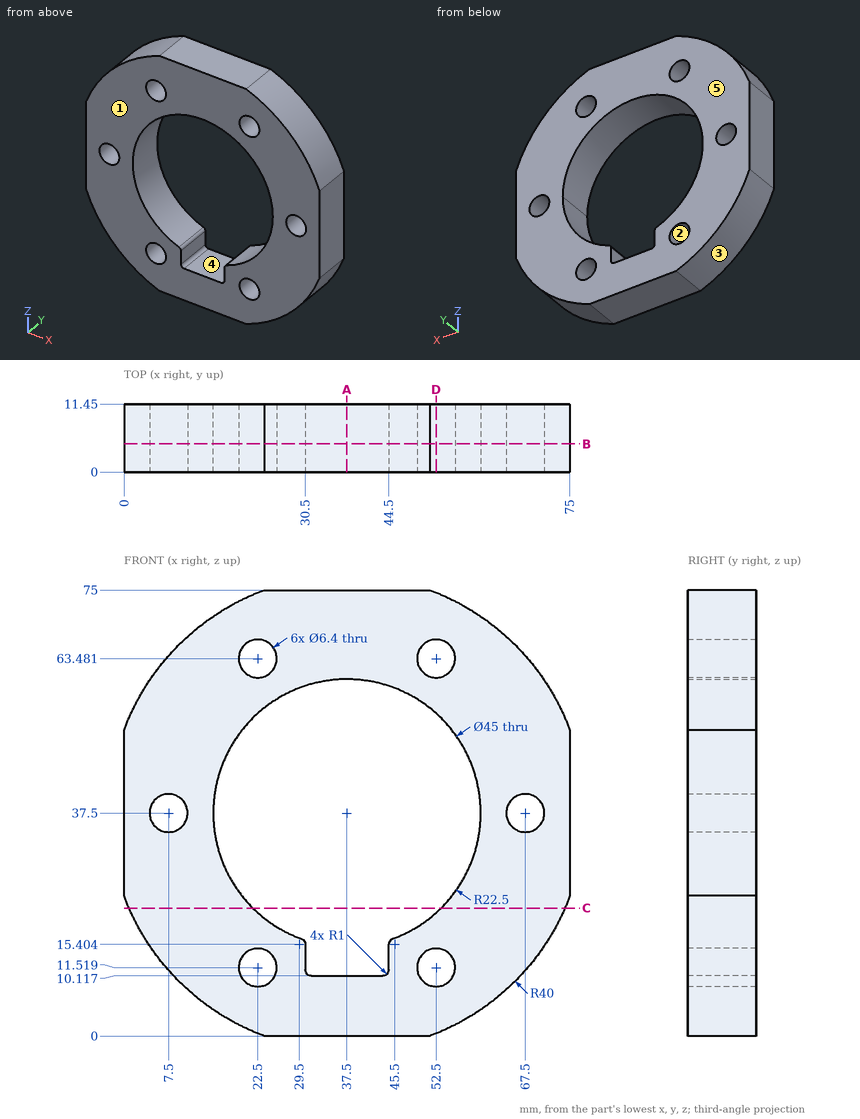
Source: three-view drawing plus pictorial views. Frame: mm from the lowest corner of the part. A direction names the side the tool comes from. Coordinates: 2 decimals unless noted, no trailing zeros. Loops run counter-clockwise (first coordinate to the right, second up) from the corner with the lowest first, then second, coordinate; pieces in that order, holes last. Notation, with made-up numbers: (42, -16) -> (68, -16) arc R13 cw to (68, 4) -> close; hole circle Ø10 at (64.25, 70). An arc over 180 degrees is marked (long way). Answer in a Markdown table with one row per item. Add a question column.
Q1. Ray query, line 1 along X through (y, z) = (2.5, 37.5); line 2 along X through (y, z) = (7.5, 61); line 3 along X through (y, z) = (1, 62) (1 decimal). Return the intervals inside material, ascending.
Q2. Section B-B on y = 4.75. Return the cut outline in (x, z), and give its area (3 significant figures).
Q3. Section C-C on z = 21.5. Return the cut outline in (x, y).
Q4. Section D-D on x = 52.5. Return the cut outline in (y, z).
Q5. Pull-direction query (Z, two-part tool) for the marked faces 1, 2 and 3; classes: pulls with the +Z half, pulls with the -Z half, needs draft (parallel to the pull), parting line crosses it, or undercut.
Q6. Reachability of the marked faces 4 and 5 from +Z, -Z, +X, -X, +Y, -Y: full face, straight path, thin tool, end or side. Return the list, or none.
Q7. Section A-A on x = 37.5. Return the cut outline in (y, z).
Q8. Contact query for flat-ended pins moving along their axis: pin 1 Ø1.5 at (y, z) = (7, 64) entering from -X; pin 2 Ø2 at (y, z) = (4, 13.5) entering from +X (1 decimal); pin 3 Ø7.5 at (x, z) = (7.5, 37.5) entering from +Y; pin 4 Ø3.5 at (y, z) = (8, 13.5) entering from -X. Output: stop coordinate, or through.
Computed values:
| question | item | result |
|---|---|---|
| 1 | line 1 | x = 0 to 4.3, 10.7 to 15, 60 to 64.3, 70.7 to 75 |
| 1 | line 2 | x = 5.13 to 20.48, 24.52 to 50.48, 54.52 to 69.87 |
| 1 | line 3 | x = 5.9 to 19.7, 25.3 to 49.7, 55.3 to 69.1 |
| 2 | outline | (0, 23.58) arc R40 ccw to (23.58, 0) -> (51.42, 0) arc R40 ccw to (75, 23.58) -> (75, 51.42) arc R40 ccw to (51.42, 75) -> (23.58, 75) arc R40 ccw to (0, 51.42) -> close; hole circle Ø6.4 at (7.5, 37.5); hole circle Ø6.4 at (22.5, 11.52); hole circle Ø6.4 at (22.5, 63.48); hole (29.84, 16.34) arc R1 cw to (30.5, 15.4) -> (30.5, 11.12) arc R1 ccw to (31.5, 10.12) -> (43.5, 10.12) arc R1 ccw to (44.5, 11.12) -> (44.5, 15.4) arc R1 cw to (45.16, 16.34) arc R22.5 ccw (long way) to start; hole circle Ø6.4 at (52.5, 11.52); hole circle Ø6.4 at (52.5, 63.48); hole circle Ø6.4 at (67.5, 37.5) |
| 2 | area | 2,980 mm^2 |
| 3 | outline | (0.84, 0) -> (21.68, 0) -> (21.68, 11.45) -> (0.84, 11.45) -> close; (53.32, 0) -> (74.16, 0) -> (74.16, 11.45) -> (53.32, 11.45) -> close |
| 4 | outline | (0, 0.42) -> (11.45, 0.42) -> (11.45, 8.32) -> (0, 8.32) -> close; (0, 14.72) -> (11.45, 14.72) -> (11.45, 20.73) -> (0, 20.73) -> close; (0, 54.27) -> (11.45, 54.27) -> (11.45, 60.28) -> (0, 60.28) -> close; (0, 66.68) -> (11.45, 66.68) -> (11.45, 74.58) -> (0, 74.58) -> close |
| 5 | face 1 | needs draft |
| 5 | face 2 | undercut |
| 5 | face 3 | pulls with the -Z half |
| 6 | face 4 | +Y, -Y |
| 6 | face 5 | +Z, -Z, +X, -X, +Y |
| 7 | outline | (0, 0) -> (11.45, 0) -> (11.45, 10.12) -> (0, 10.12) -> close; (0, 60) -> (11.45, 60) -> (11.45, 75) -> (0, 75) -> close |
| 8 | pin 1 | stops at x = 6.89 |
| 8 | pin 2 | stops at x = 70.2 |
| 8 | pin 3 | stops at y = 11.45 |
| 8 | pin 4 | stops at x = 4.26 |
